Source: three-view drawing plus pictorial views. Frame: mm from the lowest corner of the part. Coordinates: 2 decimals unless noted, no trailing zeros. Write each loop counter-clockwise with the first axis right and the second up, starting at its lowest first coordinate (ties: lowest second). Pieces come first, ordered by that corner, then holes. Notation, with made-up numbers: (60.5, 77) -> (72.5, 77) arc R30 ccw to (72.5, 112) -> close; hole circle Ø7 at (-11, -29). An arc over 180 degrees is marked (long way). One line per item, written item: value.
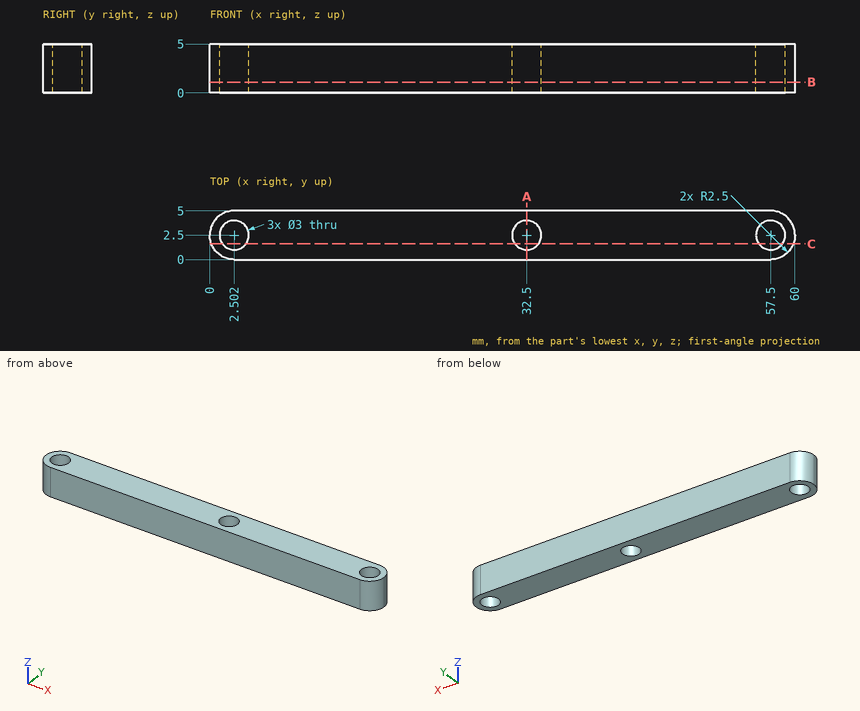
(1) Section A-A (x = 32.5). Return the cut outline in (y, z), then the cut area to 3 significant figures.
Responses:
outline: (0, 0) -> (1, 0) -> (1, 5) -> (0, 5) -> close; (4, 0) -> (5, 0) -> (5, 5) -> (4, 5) -> close
area: 10.0 mm2
(2) Section C-C (y = 1.6). Return the cut outline in (x, z), then the cut area to 3 significant figures.
Responses:
outline: (0.17, 0) -> (1.3, 0) -> (1.3, 5) -> (0.17, 5) -> close; (3.7, 0) -> (31.3, 0) -> (31.3, 5) -> (3.7, 5) -> close; (33.7, 0) -> (56.3, 0) -> (56.3, 5) -> (33.7, 5) -> close; (58.7, 0) -> (59.83, 0) -> (59.83, 5) -> (58.7, 5) -> close
area: 262 mm2
(3) Section B-B (z = 1.1). State how many separate pieces and enclosed holes the cut face has.
Responses:
separate pieces: 1
enclosed holes: 3
(4) First-contact query: pin 1 (2.5 mm diameter, centred on x = 32.5, y = 2.5, fed in from +Z). Flat tip, straight axial feed; report the tip coordinate or a pass-through.
Responses:
pin 1: passes through
(5) Line query: line 1 (X direction, y = 2.65, z = 1.1) (1 decimal); line 2 (Y direction, x = 57.5, z = 1.7); line 3 (X direction, y = 2.95, z = 0.6). Output: solid intervals per line, ascending. Write a range as [from, to].
Responses:
line 1: x = [0, 1], [4, 31], [34, 56], [59, 60]
line 2: y = [0, 1], [4, 5]
line 3: x = [0.04, 1.07], [3.93, 31.07], [33.93, 56.07], [58.93, 59.96]
